Could you check a few things on this model? Use its own coordinates, in mm. A direction names the side the tool comes from. Coordinates: 2 decimals unless noted, no trailing zeros. Loops run counter-clockwise (first coordinate to the right, second up) from the corner with the lowest first, then second, coordinate; pieces in that order, holes last. Notation, with made-up numbers: (43, 53) -> (100, 53) arc R36 ccw to (100, 91) -> close; hole circle Ø4 at (-19, 25.5). An arc over 180 degrees is marked (long way). One line per question, with ' | ' between items. Start each with the question number.
(1) Suppose I cut it at C-C (x = 6). Please give me the cut outline in (y, z).
(2) I'm going to push flat-ended pins straight in: pin 1 Ø5 at (x, z) = (4, 6) entering from -Y; pin 2 Ø1.1 at (x, z) = (-12, 5.5) entering from +Y. Where does each tip first touch, or does it pass through?
(3) Suppose I cut it at B-B (x = -15.5). Please give me the cut outline in (y, z), plus the area to 3 significant figures.
(4) Suppose I cut it at A-A (z = 13). Please give me the cut outline in (x, y).
(5) If we mould it in two halves opening along X, with no side actions, what happens to faces 4 (the face through (16.178, -4.735, 7.395)), 5 (the face through (16.309, -2.286, 7.395)), 6 (the face through (-0.3, -3.5, 15)), 7 (the face through (-17.833, -4.629, 7.395))? For each: pulls with the +X half, pulls with the -X half, needs draft (parallel to the pull), parting line crosses it, or undercut.
(6) Which directions (+Z, -Z, +X, -X, +Y, -Y) give clear straight access to the entire face, cutting with the end or side of a thin tool? Please do faces 1 (the face through (17.5, -5.2, 7.4)), 2 (the face through (11.93, -4.35, 7.4)), 3 (the face through (13.9, -3.7, 7.4)).
(7) If I drill on line 1 along X through (y, z) = (-2.2, 13.25); line 2 along X through (y, z) = (-2.75, 9.75); line 3 along X through (y, z) = (-4.7, 13.75), over which ranges is the centre line in solid material (lowest first)?
```python
from build123d import *

# Parameters (mm, degrees)
F1_DEPTH = 15


with BuildPart() as f1:
    # F0 (on Top) → F1 (new body)
    with BuildSketch(Plane.XY):
        with BuildLine():
            Line((11.5, -2), (-6, -2))
            ThreePointArc((-6, -2), (-7.118034, -2.263932), (-8, -3))
            ThreePointArc((-8, -3), (-8.881966, -3.736068), (-10, -4))
            Line((-10, -4), (-13.781936, -4))
            ThreePointArc((-13.781936, -4), (-14.249819, -4.128131), (-14.587137, -4.476769))
            Line((-14.587137, -4.476769), (-14.75, -4.661438))
            ThreePointArc((-14.75, -4.661438), (-16.161438, -4.75), (-16.25, -3.338562))
            ThreePointArc((-16.25, -3.338562), (-16.297339, -2.296813), (-17.340101, -2.308184))
            ThreePointArc((-17.340101, -2.308184), (-17.819996, -4.662142), (-15.824614, -6))
            Line((-15.824614, -6), (-9.711234, -6))
            ThreePointArc((-9.711234, -6), (-8.5932, -5.736068), (-7.711234, -5))
            ThreePointArc((-7.711234, -5), (-6.829268, -4.263932), (-5.711234, -4))
            Line((-5.711234, -4), (9.466364, -4))
            ThreePointArc((9.466364, -4), (11.959979, -4.356858), (14.253416, -5.398784))
            Line((14.253416, -5.398784), (14.663239, -5.660644))
            ThreePointArc((14.663239, -5.660644), (17.510169, -5.188916), (17.340101, -2.308184))
            ThreePointArc((17.340101, -2.308184), (16.297339, -2.296813), (16.25, -3.338562))
            ThreePointArc((16.25, -3.338562), (16.161438, -4.75), (14.75, -4.661438))
            Line((14.75, -4.661438), (13, -2.677124))
            ThreePointArc((13, -2.677124), (12.322876, -2.177124), (11.5, -2))
        make_face()
    extrude(amount=F1_DEPTH)


solid = f1.part
```
Checks:
1) outline: (-4, 0) -> (-2, 0) -> (-2, 15) -> (-4, 15) -> close
2) pin 1: stops at y = -4 | pin 2: stops at y = -4
3) outline: (-6, 0) -> (-5, 0) -> (-5, 15) -> (-6, 15) -> close | area: 15.0 mm^2
4) outline: (-17.34, -2.31) arc R2.16 ccw to (-15.82, -6) -> (-9.71, -6) arc R2.5 ccw to (-7.71, -5) arc R2.5 cw to (-5.71, -4) -> (9.47, -4) arc R8.89 cw to (14.25, -5.4) -> (14.66, -5.66) arc R2.16 ccw to (17.34, -2.31) arc R0.75 ccw to (16.25, -3.34) arc R1 cw to (14.75, -4.66) -> (13, -2.68) arc R2 ccw to (11.5, -2) -> (-6, -2) arc R2.5 ccw to (-8, -3) arc R2.5 cw to (-10, -4) -> (-13.78, -4) arc R0.92 ccw to (-14.59, -4.48) -> (-14.75, -4.66) arc R1 cw to (-16.25, -3.34) arc R0.75 ccw to start
5) face 4: undercut | face 5: undercut | face 6: needs draft | face 7: pulls with the -X half
6) face 1: +Z, -Z | face 2: +Z, -Z, -Y | face 3: +Z, -Z, +Y
7) line 1: x = -17.2 to -16.42, -6.98 to 12.37, 16.42 to 17.2 | line 2: x = -17.68 to -16.07, -7.79 to 13.06, 16.07 to 17.68 | line 3: x = -17.8 to -16.21, -14.79 to -7.45, 12.92 to 14.79, 16.21 to 17.8
